Geometry check sheet. Reference: the model listing, model coordinates, mm. A direction names the side the tool comes from. Round coordinates to 2 decimals unless told otherwise and drop trailing zeros. Write each loop counter-clockwise with the first axis right and the second up, starting at its lowest first coordinate (ties: lowest second). Pieces come first, ordered by that corner, then holes. Notation, with made-up numbers: M 6,25.25 L 50,25.25 A15 ccw 50,46.25 Z; hole C -39,28 d8. An arc over 180 degrees is marked long. Use a Markdown table: item, result.
```python
from build123d import *

# Parameters (mm, degrees)
F0_W                  = 34.2
F0_H                  = 34.2
F0_W_2                = 28.2
F0_H_2                = 28.2
F1_DEPTH              = 3
F2_DEPTH              = 31.2
F3_W                  = 34.2
F3_H                  = 34.2
F3_W_2                = 28.2
F3_H_2                = 28.2
F4_DEPTH              = 31.2
F5_W                  = 34.2
F5_H                  = 34.2
F5_W_2                = 28.2
F5_H_2                = 28.2
F6_DEPTH              = 31.2
F7_D                  = 3.3
F7_DEPTH              = 13.5
F7_CSINK_D            = 6.72
F7_CSINK_ANGLE        = 90
F7_TIP                = 0.9914200214
F7_ON_F5_D            = 3.3
F7_ON_F5_DEPTH        = 13.5
F7_ON_F5_CSINK_D      = 6.72
F7_ON_F5_CSINK_ANGLE  = 90
F7_ON_F5_TIP          = 0.9914200214
F7_ON_F3_D            = 3.3
F7_ON_F3_DEPTH        = 13.5
F7_ON_F3_CSINK_D      = 6.72
F7_ON_F3_CSINK_ANGLE  = 90
F7_ON_F3_TIP          = 0.9914200214
F8_R                  = 1.49999
F11_D                 = 3.3
F11_DEPTH             = 13.5
F11_CSINK_D           = 6.72
F11_CSINK_ANGLE       = 90
F11_TIP               = 0.9914200214
F11_ON_F9_D           = 3.3
F11_ON_F9_DEPTH       = 13.5
F11_ON_F9_CSINK_D     = 6.72
F11_ON_F9_CSINK_ANGLE = 90
F11_ON_F9_TIP         = 0.9914200214


# Not quite as in the source:
# - a fillet or chamfer is up to 0.001 mm smaller than in the source, because OpenCascade refuses the exact size


with BuildPart() as f1:
    # F0 (on Top) → F1 (new body)
    with BuildSketch(Plane.XY):
        with Locations((-14.1, 14.1)):
            Rectangle(F0_W, F0_H)
        with Locations((-14.1, 14.1)):
            Rectangle(F0_W_2, F0_H_2, mode=Mode.SUBTRACT)
        with Locations((-14.1, 14.1)):
            Rectangle(F0_W_2, F0_H_2)
    extrude(amount=-F1_DEPTH)

    # F0 (on Top) → F2 (join)
    with BuildSketch(Plane.XY):
        with Locations((-14.1, 14.1)):
            Rectangle(F0_W, F0_H)
        with Locations((-14.1, 14.1)):
            Rectangle(F0_W_2, F0_H_2, mode=Mode.SUBTRACT)
    extrude(amount=F2_DEPTH)

    # F3 (on face) → F4 (join)
    with BuildSketch(Plane.XZ.offset(3)):
        with Locations((-14.1, 14.1)):
            Rectangle(F3_W, F3_H)
        with Locations((-14.1, 14.1)):
            Rectangle(F3_W_2, F3_H_2, mode=Mode.SUBTRACT)
    extrude(amount=F4_DEPTH)

    # F5 (on face) → F6 (join)
    with BuildSketch(Plane.YZ.offset(3)):
        with Locations((14.1, 14.1)):
            Rectangle(F5_W, F5_H)
        with Locations((14.1, 14.1)):
            Rectangle(F5_W_2, F5_H_2, mode=Mode.SUBTRACT)
    extrude(amount=F6_DEPTH)

    # F7
    with Locations(Plane.XY):
        with Locations((-14.1, 14.1)):
            CounterSinkHole(F7_D / 2, F7_CSINK_D / 2, depth=F7_DEPTH, counter_sink_angle=F7_CSINK_ANGLE)
            with Locations((0, 0, -(F7_DEPTH + F7_TIP / 2))):  # 118° drill point
                Cone(0, F7_D / 2, F7_TIP, mode=Mode.SUBTRACT)

    # F7 on F5
    with Locations(Plane.YZ.offset(3)):
        with Locations((14.1, 14.1)):
            CounterSinkHole(F7_ON_F5_D / 2, F7_ON_F5_CSINK_D / 2, depth=F7_ON_F5_DEPTH, counter_sink_angle=F7_ON_F5_CSINK_ANGLE)
            with Locations((0, 0, -(F7_ON_F5_DEPTH + F7_ON_F5_TIP / 2))):  # 118° drill point
                Cone(0, F7_ON_F5_D / 2, F7_ON_F5_TIP, mode=Mode.SUBTRACT)

    # F7 on F3
    with Locations(Plane.XZ.offset(3)):
        with Locations((-14.1, 14.1)):
            CounterSinkHole(F7_ON_F3_D / 2, F7_ON_F3_CSINK_D / 2, depth=F7_ON_F3_DEPTH, counter_sink_angle=F7_ON_F3_CSINK_ANGLE)
            with Locations((0, 0, -(F7_ON_F3_DEPTH + F7_ON_F3_TIP / 2))):  # 118° drill point
                Cone(0, F7_ON_F3_D / 2, F7_ON_F3_TIP, mode=Mode.SUBTRACT)

    # F8 (radius 1.5 in the source; OpenCascade refuses exactly that, so slightly less here)
    f8_edges = [f1.edges().sort_by_distance(p)[0] for p in [
        (-31.2, -1.5, 31.2),
        (1.5, 31.2, 31.2),
        (34.2, 14.1, 31.2),
        (18.6, -3, 31.2),
        (3, -18.6, 31.2),
        (-14.1, -34.2, 31.2),
        (-14.1, 0, 31.2),
        (0, 14.1, 31.2),
        (-28.2, 14.1, 31.2),
        (-14.1, 28.2, 31.2),
        (18.6, -3, -3),
        (3, -18.6, -3),
        (-14.1, -34.2, -3),
        (-31.2, -1.5, -3),
        (1.5, 31.2, -3),
        (34.2, 14.1, -3),
        (3, -34.2, 14.1),
        (0, -34.2, 14.1),
        (-28.2, -34.2, 14.1),
        (-31.2, -34.2, 14.1),
        (-14.1, -34.2, 28.2),
        (-14.1, -34.2, 0),
        (-31.2, 31.2, 14.1),
        (34.2, 31.2, 14.1),
        (34.2, 28.2, 14.1),
        (34.2, 0, 14.1),
        (34.2, -3, 14.1),
        (34.2, 14.1, 0),
        (34.2, 14.1, 28.2),
    ]]
    fillet(f8_edges, radius=F8_R)

    # F11
    with Locations(Plane.XZ.offset(3)):
        with Locations((17.85, 14.1)):
            CounterSinkHole(F11_D / 2, F11_CSINK_D / 2, depth=F11_DEPTH, counter_sink_angle=F11_CSINK_ANGLE)
            with Locations((0, 0, -(F11_DEPTH + F11_TIP / 2))):  # 118° drill point
                Cone(0, F11_D / 2, F11_TIP, mode=Mode.SUBTRACT)

    # F11 on F9
    with Locations(Plane.YZ.offset(3)):
        with Locations((-17.85, 14.1)):
            CounterSinkHole(F11_ON_F9_D / 2, F11_ON_F9_CSINK_D / 2, depth=F11_ON_F9_DEPTH, counter_sink_angle=F11_ON_F9_CSINK_ANGLE)
            with Locations((0, 0, -(F11_ON_F9_DEPTH + F11_ON_F9_TIP / 2))):  # 118° drill point
                Cone(0, F11_ON_F9_D / 2, F11_ON_F9_TIP, mode=Mode.SUBTRACT)


solid = f1.part
```
Item 1: Mould release check, pull along Z, two halves, no side actions. Record for faces 6 (the face through (18, 28.2, 14)), 7 (the face through (-28.65, -33.77, 14.32)), 8 (the face through (2.55, -33.77, 14.32)), 9 (the face through (-13.88, -33.77, 30.75)): +Z half, -Z half, draft (parallel to the pull), parting line (faces both ways), or undercut.
Outcome:
| item | result |
|---|---|
| face 6 | undercut |
| face 7 | undercut |
| face 8 | draft |
| face 9 | +Z half |
Item 2: Go/stop test with flat-tipped pins: pin 1 (4 mm diameter, centred on y = -9.5, z = 15.5, fed in from +X); pin 2 (3 mm diameter, centred on x = -13, y = 24.5, fed in from +Z); pin 3 (2.5 mm diameter, centred on y = -17.85, z = 14.1, fed in from +X). Record where each tip stops, or that it passes through.
Outcome:
| item | result |
|---|---|
| pin 1 | stops at x = 3 |
| pin 2 | stops at z = 0 |
| pin 3 | stops at x = -28.2 |
Item 3: Material ranges on line 1 along X through (y, z) = (4, 13); line 2 along Y through (x, z) = (-5, 12.5), recorded low to high. Write a range as from..to.
Outcome:
| item | result |
|---|---|
| line 1 | x = -31.2..-28.2, 0..3 |
| line 2 | y = -3..0, 28.2..31.2 |
Item 4: Cross-section at A-A, the plane y = 14.1. Count the separate pieces of the cut face and the enclosed holes in it, and give its area (3 significant figures).
Outcome:
| item | result |
|---|---|
| separate pieces | 3 |
| enclosed holes | 0 |
| area | 447 mm2 |
Item 5: Access from +Z, -Z, +X, -X, +Y, -Y to the whole of each face (thin tool, end or side, straight path). Record for faces 1 (the face through (2.57, -17.32, -2.55)), 2 (the face through (33.77, -0.45, 14.32)), 3 (the face through (0.43, 14.32, 30.75)), 4 (the face through (3, -14, 14)), 5 (the face through (17.32, -2.57, 30.75)).
Outcome:
| item | result |
|---|---|
| face 1 | -Z, +X, -Y |
| face 2 | +X |
| face 3 | +Z |
| face 4 | +Z, -Z, +X, -Y |
| face 5 | +Z, +X, -Y |
Item 6: Cross-section at B-B, the plane x = 10. Record the cut outline in (y, z).
Outcome:
| item | result |
|---|---|
| outline | M -3,-1.5 A1.5 ccw -1.5,-3 L 29.7,-3 A1.5 ccw 31.2,-1.5 L 31.2,29.7 A1.5 ccw 29.7,31.2 L -1.5,31.2 A1.5 ccw -3,29.7 Z; hole M 0,0 L 28.2,0 L 28.2,28.2 L 0,28.2 Z |
